Read the model definition and answer for the solid it produces. Units are mm, in the model's axes. A direction names the side the tool comes from. Round coordinates to 2 decimals unless told otherwise and drop trailing zeros. Write each loop counter-clockwise with the first axis right and the second up, starting at its lowest first coordinate (ties: lowest second). Pieces come first, ordered by that corner, then holes. Notation, with made-up numbers: (58.25, -35) - (68.25, -35) arc R11 cw to (68.25, -28) - close; hole circle Ø5 at (46.5, 80). An arc over 180 degrees is marked (long way). One line per item, written item: value. Start each with the question number.
(1) A cutting plane is placed at B-B, the plane z = 11. Determine the outline of the cut face in (x, y).
(2) Find the intervals of material crossed by L1, parallel to Z at x = -9, y = 3.25; L2, parallel to Y at x = -9, z = -32.5; L3, parallel to X at y = 17.25, z = 3, in increasing order.
(3) Flat-ended cylindrical pins translate along their axes: pin 1 Ø5.5 at (x, z) = (10.5, 47.75) entering from -Y; pin 2 Ø6 at (y, z) = (15, 27.5) entering from -X; pin 3 Ø2 at (x, y) = (-7.5, 8.5) entering from +Z; pin 4 Ø3.5 at (x, y) = (6, 9.5) entering from -Z. Find the tip coordinate at first contact, or state that the pin passes through.
(4) A cutting plane is placed at C-C, the plane x = 4.5. Determine the outline of the cut face in (y, z), plus the area to 3 significant figures.
(5) The mould has two halves that part along Z. Classify faces 4 (the face through (-25, 5, -1)), 5 (the face through (11.399, 2.465, 44.888)), 6 (the face through (50.03, 2.46, -34.86)), 7 (the face through (-50.49, 2.54, -50.72)): +Z half, -Z half, draft (parallel to the pull), parting line (faces both ways), or undercut.
(6) A cutting plane is placed at A-A, the plane x = -18. Determine the outline of the cut face in (y, z), plus the area to 3 significant figures.
(7) A cutting plane is placed at D-D, the plane z = 0. Determine the outline of the cut face in (x, y).
(8) For faces 1 (the face through (0, 8, 30)), 2 (the face through (24.86, 12.12, 1.08)), 3 (the face through (50.472, 2.465, -10.86)), determine the directions among +Z, -Z, +X, -X, +Y, -Y from which every point of the face is accessible in a straight line to the end or side of a thin tool.
from build123d import *

# Parameters (mm, degrees)
SKETCH1_W                = 110
SKETCH1_H                = 110
BOSS_EXTRUDE1_DEPTH      = 5
FILLET2_R                = 15
FILLET3_R                = 15
FILLET4_R                = 15
FILLET5_R                = 15
SKETCH2_W                = 30
SKETCH2_H                = 60
BOSS_EXTRUDE2_DEPTH      = 24
BOSS_EXTRUDE3_DEPTH      = 20
BOSS_EXTRUDE3_DEPTH_BACK = 50
SKETCH4_R                = 5
FILLET6_R                = 10
FILLET7_R                = 10
SKETCH5_R                = 3
CUT_EXTRUDE2_DEPTH       = 10
CUT_EXTRUDE3_DEPTH       = 60


with BuildPart() as part:
    # Sketch1 → Boss-Extrude1 (new body)
    with BuildSketch(Plane(origin=(0, 0, 0), x_dir=(1, 0, 0), z_dir=(0, 1, 0))):
        Rectangle(SKETCH1_W, SKETCH1_H)
    extrude(amount=BOSS_EXTRUDE1_DEPTH)

    # Fillet2
    fillet2_edges = [part.edges().sort_by_distance(p)[0] for p in [
        (55, 2.5, -55),
    ]]
    fillet(fillet2_edges, radius=FILLET2_R)

    # Fillet3
    fillet3_edges = [part.edges().sort_by_distance(p)[0] for p in [
        (-55, 2.5, -55),
    ]]
    fillet(fillet3_edges, radius=FILLET3_R)

    # Fillet4
    fillet4_edges = [part.edges().sort_by_distance(p)[0] for p in [
        (-55, 2.5, 55),
    ]]
    fillet(fillet4_edges, radius=FILLET4_R)

    # Fillet5
    fillet5_edges = [part.edges().sort_by_distance(p)[0] for p in [
        (55, 2.5, 55),
    ]]
    fillet(fillet5_edges, radius=FILLET5_R)

    # Sketch2 → Boss-Extrude2 (add)
    with BuildSketch(Plane(origin=(0, 5, 0), x_dir=(1, 0, 0), z_dir=(0, 1, 0))):
        Rectangle(SKETCH2_W, SKETCH2_H)
    extrude(amount=BOSS_EXTRUDE2_DEPTH)

    # Sketch4 → Boss-Extrude3 (add, two sides: drawn at the far end of the back side and taken through both)
    with BuildSketch(Plane(origin=(15, 0, 0), x_dir=(0, 0, -1), z_dir=(1, 0, 0)).offset(-BOSS_EXTRUDE3_DEPTH_BACK)):
        with Locations((0, 17)):
            Circle(SKETCH4_R)
    extrude(amount=BOSS_EXTRUDE3_DEPTH + BOSS_EXTRUDE3_DEPTH_BACK)

    # Fillet6
    fillet6_edges = [part.edges().sort_by_distance(p)[0] for p in [
        (0, 29, 30),
    ]]
    fillet(fillet6_edges, radius=FILLET6_R)

    # Fillet7
    fillet7_edges = [part.edges().sort_by_distance(p)[0] for p in [
        (0, 29, -30),
    ]]
    fillet(fillet7_edges, radius=FILLET7_R)

    # Sketch5 → Cut-Extrude2 (cut)
    with BuildSketch(Plane.XZ):
        with Locations(Location((47.497955542, -11.251022229, 0), (0, 0, 270))):
            Circle(SKETCH5_R)
        with Locations(Location((47.497955542, 32.748977771, 0), (0, 0, 270))):
            Circle(SKETCH5_R)
        with Locations(Location((-48.502044458, 10.748977771, 0), (0, 0, 270))):
            Circle(SKETCH5_R)
        with Locations(Location((-48.502044458, -11.251022229, 0), (0, 0, 270))):
            Circle(SKETCH5_R)
        with Locations(Location((-48.502044458, -33.251022229, 0), (0, 0, 270))):
            Circle(SKETCH5_R)
        with Locations(Location((-33.502044458, -48.251022229, 0), (0, 0, 270))):
            Circle(SKETCH5_R)
        with Locations(Location((-11.502044458, -48.251022229, 0), (0, 0, 270))):
            Circle(SKETCH5_R)
        with Locations(Location((10.497955542, -48.251022229, 0), (0, 0, 270))):
            Circle(SKETCH5_R)
        with Locations(Location((32.497955542, -48.251022229, 0), (0, 0, 270))):
            Circle(SKETCH5_R)
        with Locations(Location((47.497955542, -33.251022229, 0), (0, 0, 270))):
            Circle(SKETCH5_R)
        with Locations(Location((47.497955542, 10.748977771, 0), (0, 0, 270))):
            Circle(SKETCH5_R)
        with Locations(Location((32.497955542, 47.748977771, 0), (0, 0, 270))):
            Circle(SKETCH5_R)
        with Locations(Location((10.497955542, 47.748977771, 0), (0, 0, 270))):
            Circle(SKETCH5_R)
        with Locations(Location((-11.502044458, 47.748977771, 0), (0, 0, 270))):
            Circle(SKETCH5_R)
        with Locations(Location((-33.502044458, 47.748977771, 0), (0, 0, 270))):
            Circle(SKETCH5_R)
        with Locations(Location((-48.502044458, 32.748977771, 0), (0, 0, 270))):
            Circle(SKETCH5_R)
    extrude(amount=-CUT_EXTRUDE2_DEPTH, mode=Mode.SUBTRACT)

    # Sketch8 → Cut-Extrude3 (cut)
    with BuildSketch(Plane.ZY.offset(15)):
        with BuildLine():
            Line((-30, 19), (-30, 12))
            ThreePointArc((-30, 12), (0, 24.426406871), (30, 12))
            Line((30, 12), (30, 19))
            ThreePointArc((30, 19), (27.071067812, 26.071067812), (20, 29))
            Line((20, 29), (-20, 29))
            ThreePointArc((-20, 29), (-27.071067812, 26.071067812), (-30, 19))
        make_face()
    extrude(amount=-CUT_EXTRUDE3_DEPTH, mode=Mode.SUBTRACT)


solid = part.part
Here are the results:
1. outline: (-55, 0) - (-51.49, 0) - (-51.49, 5) - (-55, 5) - close; (-45.51, 0) - (44.51, 0) - (44.51, 5) - (15, 5) - (15, 22.98) - (-15, 22.98) - (-15, 5) - (-45.51, 5) - close; (50.49, 0) - (55, 0) - (55, 5) - (50.49, 5) - close
2. L1: -55 to -49.91, -46.6 to 46.09, 49.4 to 55
2. L2: 0 to 5
2. L3: -35 to 35
3. pin 1: through
3. pin 2: x = -15
3. pin 3: z = 30
3. pin 4: z = -30
4. outline: (0, -55) - (5, -55) - (5, -30) - (12, -30) arc R42.43 ccw to (12, 30) - (5, 30) - (5, 55) - (0, 55) - close
4. area: 1,480 mm²
5. face 4: draft
5. face 5: undercut
5. face 6: undercut
5. face 7: -Z half
6. outline: (0, -55) - (5, -55) - (5, 55) - (0, 55) - close; circle Ø10 at (17, 0)
6. area: 629 mm²
7. outline: (-55, 0) - (55, 0) - (55, 5) - (15, 5) - (15, 12) - (35, 12) - (35, 22) - (15, 22) - (15, 24.43) - (-15, 24.43) - (-15, 22) - (-35, 22) - (-35, 12) - (-15, 12) - (-15, 5) - (-55, 5) - close
8. face 1: +Z, +X, -X, +Y
8. face 2: +X
8. face 3: +Y, -Y
